For this review, take the finished solid that the model builds, in its own axes (mm). A direction names the side the tool comes from. Coordinates: 2 decimals unless noted, no trailing zeros. Write each loop counter-clockwise with the first axis right and the second up, starting at its lowest first coordinate (ties: lowest second). Pieces come first, ordered by that corner, then holes. Notation, with made-up numbers: M 44.5,66.5 L 61.5,66.5 A21 cw 61.5,92.5 Z; hole C 81.25,59.25 d1. An arc over 180 degrees is marked long. Return JSON: item names as keys, results as strings.
```python
from build123d import *

# Parameters (mm, degrees)
SKETCH1_W               = 91.44
SKETCH1_H               = 71.374
BOSS_EXTRUDE1_DEPTH     = 103.378
BOSS_EXTRUDE2_DEPTH     = 91.44
SKETCH3_W               = 6.35
SKETCH3_H               = 8.525765965
SKETCH3_W_2             = 63.5
CUT_EXTRUDE1_DEPTH      = 162.17684191
FILLET1_R               = 2.54
CUT_EXTRUDE2_DEPTH      = 162.176841809
CUT_EXTRUDE2_DEPTH_BACK = 162.176841809
SKETCH4_R               = 1.27
SKETCH5_R               = 1.27
CUT_EXTRUDE3_DEPTH      = 162.176841809


with BuildPart() as part:
    # Sketch1 → Boss-Extrude1 (new body)
    with BuildSketch(Plane(origin=(0, 0, 0), x_dir=(1, 0, 0), z_dir=(0, 1, 0))):
        with Locations((45.72, 35.687)):
            Rectangle(SKETCH1_W, SKETCH1_H)
    extrude(amount=BOSS_EXTRUDE1_DEPTH)

    # Sketch2 → Boss-Extrude2 (add)
    with BuildSketch(Plane(origin=(91.44, 0, 0), x_dir=(0, 0, -1), z_dir=(1, 0, 0))):
        with BuildLine():
            Line((12.671032171, 103.378), (14.576032171, 103.378))
            add(Edge.make_bspline(
                [(14.576032171, 103.378), (14.461628567, 108.255817866), (18.882181929, 109.998765965)],
                knots=[0, 0, 0, 1, 1, 1], degree=2))
            Line((18.882181929, 109.998765965), (18.882181929, 111.903765965))
            add(Edge.make_bspline(
                [(12.671032171, 103.378), (12.919876826, 109.602255935), (18.882181929, 111.903765965)],
                knots=[0, 0, 0, 1, 1, 1], degree=2))
        make_face()
    extrude(amount=-BOSS_EXTRUDE2_DEPTH)

    # Sketch3 → Cut-Extrude1 (cut, through all)
    with BuildSketch(Plane.XY):
        with Locations((3.175, 107.640882983)):
            Rectangle(SKETCH3_W, SKETCH3_H)
        with Locations((45.72, 107.640882983)):
            Rectangle(SKETCH3_W_2, SKETCH3_H)
        with Locations((88.265, 107.640882983)):
            Rectangle(SKETCH3_W, SKETCH3_H)
    extrude(amount=-CUT_EXTRUDE1_DEPTH, mode=Mode.SUBTRACT)

    # Fillet1
    fillet1_edges = [part.edges().sort_by_distance(p)[0] for p in [
        (91.44, 103.378, -35.687),
        (45.72, 103.378, -71.374),
        (0, 103.378, -35.687),
        (45.72, 103.378, 0),
    ]]
    fillet(fillet1_edges, radius=FILLET1_R)

    # Sketch4 → Cut-Extrude2 (cut, two sides: drawn at the far end of the back side and taken through both)
    with BuildSketch(Plane.ZY.offset(-CUT_EXTRUDE2_DEPTH_BACK)):
        with Locations((-71.374, 80.518)):
            Circle(SKETCH4_R)
        with Locations((0, 80.518)):
            Circle(SKETCH4_R)
    extrude(amount=CUT_EXTRUDE2_DEPTH + CUT_EXTRUDE2_DEPTH_BACK, mode=Mode.SUBTRACT)

    # Sketch5 → Cut-Extrude3 (cut, through all)
    with BuildSketch(Plane.XY):
        with Locations((0, 80.518)):
            Circle(SKETCH5_R)
        with Locations((91.44, 80.518)):
            Circle(SKETCH5_R)
    extrude(amount=-CUT_EXTRUDE3_DEPTH, mode=Mode.SUBTRACT)


solid = part.part
```
1. We need section A-A (z = -10.5). State the section outline as (x, y) points.
Checks:
{"outline": "M 0,0 L 91.44,0 L 91.44,79.25 A1.27 cw 91.44,81.79 L 91.44,100.84 A2.54 ccw 88.9,103.38 L 2.54,103.38 A2.54 ccw 0,100.84 L 0,81.79 A1.27 cw 0,79.25 Z"}
2. Clearance check with flat-ended pins moving along their axes: pin 1 Ø10 at (x, z) = (32.5, -50.5) entering from +Y; pin 2 Ø5 at (y, z) = (109, -17) entering from +X; pin 3 Ø3 at (y, z) = (107, -15.5) entering from -X. State where each tip first meets the part, or that it passes through.
Checks:
{"pin 1": "y = 103.38", "pin 2": "x = 85.09", "pin 3": "x = 6.35"}
3. Wall thickness on L1, parallel to Y at x = 61.5, z = -12: over which ranges is the line inside the solid? List them lowest first. Write a range as from..to.
Checks:
{"L1": "0..103.38"}
4. Draft analysis for pull direction Y (two halves, no side actions). For faces 1 (the face through (85.09, 108, -15)), 2 (the face through (0.72, 102.61, -36.19)), 3 (the face through (46.36, 80.49, -70.104)), state which applies: +Y half, -Y half, draft (parallel to the pull), parting line (faces both ways), or undercut.
Checks:
{"face 1": "draft", "face 2": "+Y half", "face 3": "undercut"}
5. For faces 4 (the face through (77.47, 108, -15)), 5 (the face through (45, 39, -71.374)), 6 (the face through (6.35, 108, -15)), list the 3-axis set-ups (+Z, -Z, +X, -X, +Y, -Y) from which the entire face can be reached by the end or side of a thin tool; tool diameter is ignored.
Checks:
{"face 4": "+Z, -Z, +Y", "face 5": "-Z, +X, -X, +Y, -Y", "face 6": "+Z, -Z, -X, +Y"}
6. We need section B-B (x = 66). State the section outline as (y, z) points, plus the area to 3 significant figures.
Checks:
{"outline": "M 0,-71.37 L 79.25,-71.37 A1.27 cw 81.79,-71.37 L 100.84,-71.37 A2.54 ccw 103.38,-68.83 L 103.38,-2.54 A2.54 ccw 100.84,0 L 81.79,0 A1.27 cw 79.25,0 L 0,0 Z", "area": "7,370 mm2"}
